```python
from build123d import *

# Parameters (mm, degrees)
RESSALTO_EXTRUS_O1_DEPTH = 5
RESSALTO_EXTRUS_O2_DEPTH = 31
ESBO_O3_R                = 1.38
CORTE_EXTRUS_O1_DEPTH    = 5
CORTE_EXTRUS_O2_DEPTH    = 5


with BuildPart() as part:
    # Esboço1 → Ressalto-extrusão1 (new body)
    with BuildSketch(Plane.XY):
        with BuildLine():
            Line((-78, -61.175), (78, -61.175))
            ThreePointArc((78, -61.175), (80.5, -58.675), (78, -56.175))
            ThreePointArc((78, -56.175), (75.75493597, -50.75493597), (81.175, -53))
            ThreePointArc((81.175, -53), (83.675, -55.5), (86.175, -53))
            Line((86.175, -53), (86.175, 53))
            ThreePointArc((86.175, 53), (83.675, 55.5), (81.175, 53))
            ThreePointArc((81.175, 53), (75.756150129, 50.753722467), (77.996566768, 56.174998144))
            ThreePointArc((77.996566768, 56.174998144), (80.493861975, 58.677700014), (77.991160104, 61.174995221))
            Line((77.991160104, 61.174995221), (-78, 61.174995221))
            ThreePointArc((-78, 61.174995221), (-80.5, 58.674995221), (-78, 56.174995221))
            ThreePointArc((-78, 56.174995221), (-75.75493597, 50.75493119), (-81.175, 52.999995221))
            ThreePointArc((-81.175, 52.999995221), (-83.675, 55.499995221), (-86.175, 52.999995221))
            Line((-86.175, 52.999995221), (-86.175, -53))
            ThreePointArc((-86.175, -53), (-83.675, -55.5), (-81.175, -53))
            ThreePointArc((-81.175, -53), (-75.75493597, -50.75493597), (-78, -56.175))
            ThreePointArc((-78, -56.175), (-80.5, -58.675), (-78, -61.175))
        make_face()
    extrude(amount=RESSALTO_EXTRUS_O1_DEPTH)

    # Esboço2 → Ressalto-extrusão2 (add)
    with BuildSketch(Plane.XY.offset(5)):
        with BuildLine():
            Line((-78, -56.175), (-35.5, -56.175))
            Line((-35.5, -56.175), (-35.5, -60.212223694))
            Line((-35.5, -60.212223694), (-35.5, -61.175))
            Line((-35.5, -61.175), (-78, -61.175))
            ThreePointArc((-78, -61.175), (-80.5, -58.675), (-78, -56.175))
        make_face()
        with BuildLine():
            Line((78, -61.175), (65.099265532, -61.175))
            Line((65.099265532, -61.175), (65.099265532, -56.175))
            Line((65.099265532, -56.175), (78, -56.175))
            ThreePointArc((78, -56.175), (80.5, -58.675), (78, -61.175))
        make_face()
    extrude(amount=RESSALTO_EXTRUS_O2_DEPTH)

    # Esboço3 → Corte-extrusão1 (cut)
    with BuildSketch(Plane.XY.offset(5)):
        with Locations((59.125349465, -41.637776306)):
            Circle(ESBO_O3_R)
        with Locations((59.125349465, 16.362223694)):
            Circle(ESBO_O3_R)
        with Locations((-26.874650535, -41.637776306)):
            Circle(ESBO_O3_R)
        with Locations((-26.874650535, 16.362223694)):
            Circle(ESBO_O3_R)
    extrude(amount=-CORTE_EXTRUS_O1_DEPTH, mode=Mode.SUBTRACT)

    # Esboço4 → Corte-extrusão2 (cut)
    with BuildSketch(Plane.XY.offset(5)):
        with BuildLine():
            Line((-61.175, 38.825), (-51.175, 38.825))
            ThreePointArc((-51.175, 38.825), (-47.639466094, 37.360533906), (-46.175, 33.825))
            Line((-46.175, 33.825), (-46.175, -36.175))
            ThreePointArc((-46.175, -36.175), (-47.639466094, -39.710533906), (-51.175, -41.175))
            Line((-51.175, -41.175), (-61.175, -41.175))
            ThreePointArc((-61.175, -41.175), (-64.710533906, -39.710533906), (-66.175, -36.175))
            Line((-66.175, -36.175), (-66.175, 33.825))
            ThreePointArc((-66.175, 33.825), (-64.710533906, 37.360533906), (-61.175, 38.825))
        make_face()
    extrude(amount=-CORTE_EXTRUS_O2_DEPTH, mode=Mode.SUBTRACT)


solid = part.part
```
Work out the finished part from the listing and answer in its coordinate system (mm). A direction names the side the tool comes from. Round coordinates to 2 decimals unless told otherwise and drop trailing zeros. Write each loop counter-clockwise with the first axis right and the second up, starting at its lowest first coordinate (ties: lowest second). Pieces come first, ordered by that corner, then holes. Notation, with made-up numbers: (1, 30) -> (21, 30) arc R26 cw to (21, 65) -> close; hole circle Ø1 at (88.5, -15.75). An arc over 180 degrees is marked (long way). Write each question's results on one line, items separated by ' | '.
Q1. Flat-ended cylindrical pins translate along their axes: P1, Ø1.5, axis at y = -59.5, z = 27.5, coming from the -X side; P2, Ø1.5, axis at y = -59.5, z = 13.5, coming from the +X side; P3, Ø10, axis at x = 5.5, y = 15, coming from the +Z side. Find the tip coordinate at first contact, or state that the pin passes through.
Data:
P1: x = -80.5 | P2: x = 80.5 | P3: z = 5
Q2. Section A-A, the plane z = 10 is taken. Write down the section's boundary in (x, y) (3 decimals), then the cut area to 3 significant figures.
Data:
outline: (-78, -61.175) -> (-35.5, -61.175) -> (-35.5, -56.175) -> (-78, -56.175) arc R2.5 ccw to start; (65.099, -61.175) -> (78, -61.175) arc R2.5 ccw to (78, -56.175) -> (65.099, -56.175) -> close | area: 297 mm^2
Q3. Section B-B, the plane y = 29.5 is taken. Write down the section's boundary in (x, z) (3 decimals), then the cut area to 3 significant figures.
Data:
outline: (-86.175, 0) -> (-66.175, 0) -> (-66.175, 5) -> (-86.175, 5) -> close; (-46.175, 0) -> (86.175, 0) -> (86.175, 5) -> (-46.175, 5) -> close | area: 762 mm^2
Q4. Which of the six approach directions +Z, -Z, +X, -X, +Y, -Y give full straight-line access (tool end or side, diameter ignored) to faces 4 (the flat face through (65.099, -59, 20)), 5 (the flat face through (-56, 38.825, 3)), 6 (the cylindrical face through (-83.7, -55.5, 2.5))?
Data:
face 4: +Z, +Y, -Y | face 5: +Z, -Z | face 6: +Z, -Z, -Y
Q5. Straight lines are drawn through the part: line 1 along Y through (x, z) = (-78, 1.8) (3 decimals); line 2 along X through (y, z) = (53, 3.15) (3 decimals); line 3 along X through (y, z) = (-2, 3) (3 decimals). For each, find the intervals that lie inside material, in ascending order. Write a range as [from, to].
Data:
line 1: [-61.175, -56.175], [-49.825, 49.825], [56.175, 61.175] | line 2: [-86.175, -81.175], [-74.825, 74.825], [81.175, 86.175] | line 3: [-86.175, -66.175], [-46.175, 86.175]
Q6. Section C-C, the plane x = 4.5 is taken. Write down the section's boundary in (y, z) (3 decimals).
Data:
outline: (-61.175, 0) -> (61.175, 0) -> (61.175, 5) -> (-61.175, 5) -> close
Q7. Determine the mould class of faces 1 (the flat face through (-1, 1, 0)), 2 (the cylindrical face through (-75.68, 50.83, 2.46)), 3 (the flat face through (86.175, -1, 2)) for opening direction X: released by +X, released by -X, zero draft, split by the parting line, or undercut.
Data:
face 1: zero draft | face 2: undercut | face 3: released by +X
